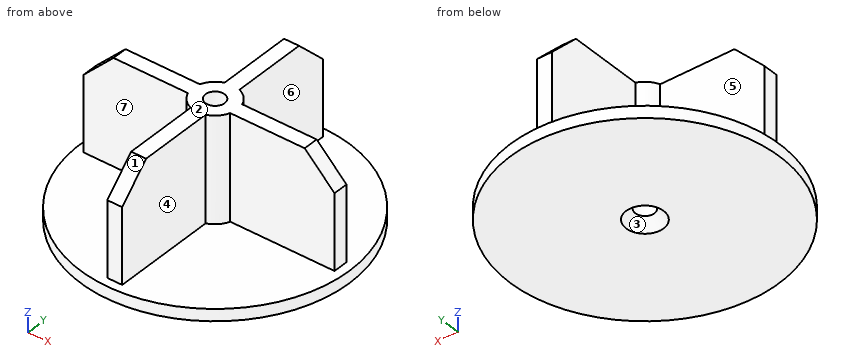
```python
from build123d import *

# Parameters (mm, degrees)
F0_R           = 28.575
F1_DEPTH       = 2.54
F3_DEPTH       = 22.352
F4_SIZE        = 6.35
F5_R           = 4.7625
F6_DEPTH       = 22.352
F8_D           = 4.064
F8_CSINK_D     = 7.9502
F8_CSINK_ANGLE = 82


with BuildPart() as f1:
    # F0 (on Top) → F1 (new body)
    with BuildSketch(Plane.XY):
        Circle(F0_R)
    extrude(amount=F1_DEPTH)

    # F2 (on face) → F3 (join)
    with BuildSketch(Plane.XY.offset(2.54)):
        Polygon((26.67, -1.5875), (26.67, 1.5875), (1.5875, 1.5875), (1.5875, 26.67), (-1.5875, 26.67), (-1.5875, 1.5875), (-26.67, 1.5875), (-26.67, -1.5875), (-1.5875, -1.5875), (-1.5875, -26.67), (1.5875, -26.67), (1.5875, -1.5875), align=None)
    extrude(amount=F3_DEPTH)

    # F4
    f4_edges = [f1.edges().sort_by_distance(p)[0] for p in [
        (0, -26.67, 24.892),
        (26.67, 0, 24.892),
        (0, 26.67, 24.892),
        (-26.67, 0, 24.892),
    ]]
    chamfer(f4_edges, length=F4_SIZE)

    # F5 (on face) → F6 (join, through all)
    with BuildSketch(Plane.XY.offset(24.892)):
        Circle(F5_R)
    extrude(amount=-F6_DEPTH)

    # F8 (through all)
    with Locations(Plane(origin=(0, 0, 0), x_dir=(1, 0, 0), z_dir=(0, 0, -1))):
        with Locations((0, 0)):
            CounterSinkHole(F8_D / 2, F8_CSINK_D / 2, counter_sink_angle=F8_CSINK_ANGLE)


solid = f1.part
```
Geometry check sheet. Reference: the model listing, model coordinates, mm. Face numbers are marked on the shaded views. A direction names the side the tool comes from. Give positions to 0.01 mm unless a question says otherwise; leave off trailing zeros. Loops run counter-clockwise (first coordinate to the right, second up) from the corner with the lowest first, then second, coordinate; pieces in that order, holes last. Notation, with made-up numbers: M 5.25,40 L 12.25,40 A20 ccw 12.25,48 Z; hole C -6.5,33 d11. An arc over 180 degrees is marked long. Write item = value, one per line. Start each with the question number.
1. Tool access check on the marked faces 4, 5, 6 and 7. Record the directions out of +Z, -Z, +X, -X, +Y, -Y that give a thin tool (end or side, any length) a straight path to the whole face; none if there is none.
2. Thickness scan on probe 1 along Y at (x, z) = (0, 18.25); probe 2 along X at (y, z) = (-15, 14.5); probe 3 along Z at (x, y) = (4.5, -7). Record the ranges inside material, lowest first.
3. Go/stop test with flat-tipped pins: P1, Ø1, axis at x = 0, z = 11, coming from the -Y side; P2, Ø8, axis at x = 22.5, z = 6, coming from the +Y side; P3, Ø12, axis at x = -12, y = -22.5, coming from the +Z side; P4, Ø2.5, axis at x = 0, y = 0, coming from the -Z side. Record where each tip stops, or that it passes through.
4. Draft check along Y on the marked faces 1, 2 and 3. Enter one of: +Y half, -Y half, draft (parallel to the pull), parting line (faces both ways), or undercut.
5. Section check A-A, the plane z = 13.5. Enter the section's corners in (x, y) (1 decimal).
6. Section check D-D, the plane x = -18.5. Enter the section's corners in (y, z).
7. Section check B-B, the plane y = 0. Enter the section's corners in (x, z) (3 decimals), plus the area to 3 significant figures.
Values follow:
q1.face_4 = +Z, +X, -Y
q1.face_5 = +Z, -X, +Y
q1.face_6 = +Z, +X, +Y
q1.face_7 = +Z, -X, -Y
q2.probe_1 = -26.67 to -2.03, 2.03 to 26.67
q2.probe_2 = -1.59 to 1.59
q2.probe_3 = 0 to 2.54
q3.P1 = -26.67
q3.P2 = 19.91
q3.P3 = 2.54
q3.P4 = through
q4.face_1 = -Y half
q4.face_2 = draft
q4.face_3 = undercut
q5.outline = M -26.7,-1.6 L -4.5,-1.6 A4.8 ccw -1.6,-4.5 L -1.6,-26.7 L 1.6,-26.7 L 1.6,-4.5 A4.8 ccw 4.5,-1.6 L 26.7,-1.6 L 26.7,1.6 L 4.5,1.6 A4.8 ccw 1.6,4.5 L 1.6,26.7 L -1.6,26.7 L -1.6,4.5 A4.8 ccw -4.5,1.6 L -26.7,1.6 Z; hole C 0,0 d4.1
q6.outline = M -21.78,0 L 21.78,0 L 21.78,2.54 L 1.59,2.54 L 1.59,24.89 L -1.59,24.89 L -1.59,2.54 L -21.78,2.54 Z
q7.outline = M -28.575,0 L -3.975,0 L -2.032,2.235 L -2.032,24.892 L -20.32,24.892 L -26.67,18.542 L -26.67,2.54 L -28.575,2.54 Z; M 2.032,2.235 L 3.975,0 L 28.575,0 L 28.575,2.54 L 26.67,2.54 L 26.67,18.542 L 20.32,24.892 L 2.032,24.892 Z
q7.area = 1,190 mm^2
